Check sheet for the drawn part. Datum: minimum x, y, z corner. Units: mm. A direction names the side the tool comes from. Round coordinates to 2 decimals unless told otherwise and drop trailing zeros. Write each loop counter-clockwise with the first axis right and the second up, starting at its lowest first coordinate (ties: lowest second). Pieces come first, ordered by that corner, then holes. Notation, with made-up numbers: (67, -29) -> (114, -29) arc R18 ccw to (114, 3) -> close; hole circle Ø7 at (86.25, -34). An arc over 180 degrees is marked (long way). Use CSV: the item, a comma, the result in double quotes.
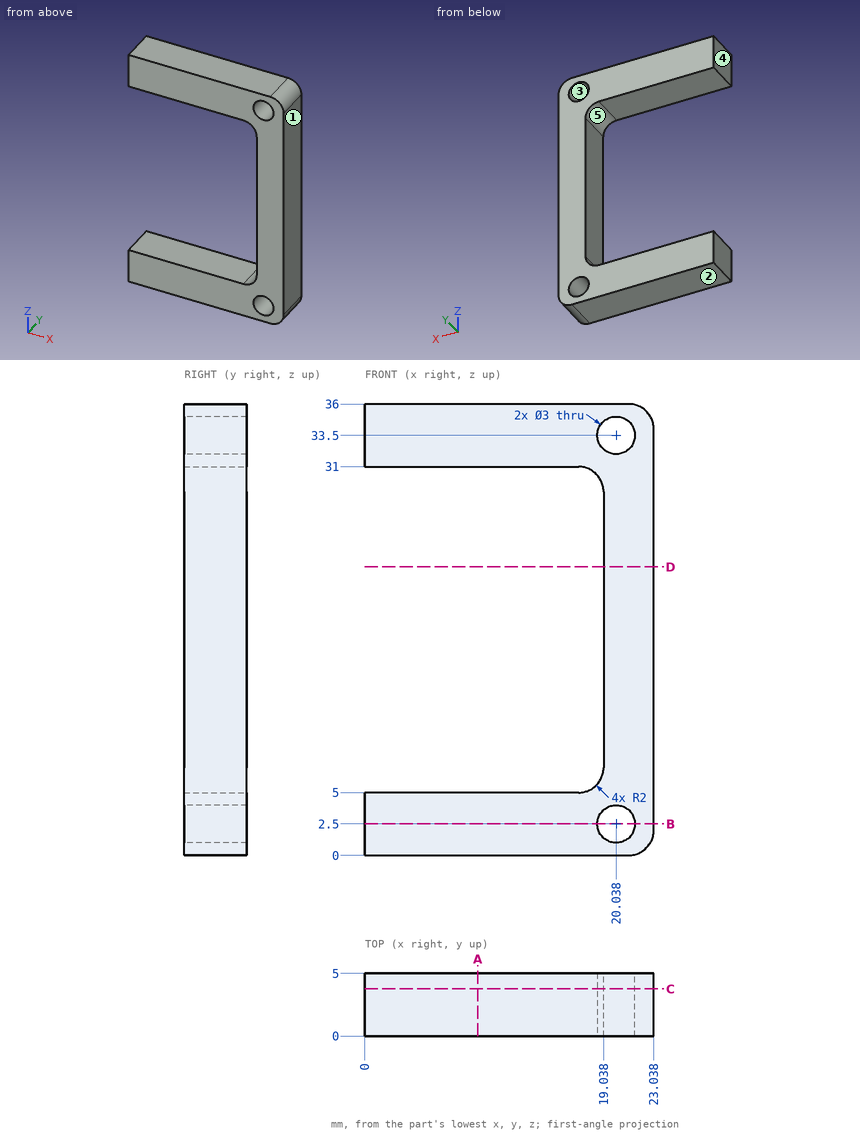
Q1. Section check B-B (z = 2.5). Record the cut outline in (x, y), plus the area to 3 significant figures.
Filled in:
outline,"(0, 0) -> (18.54, 0) -> (18.54, 5) -> (0, 5) -> close; (21.54, 0) -> (23.04, 0) -> (23.04, 5) -> (21.54, 5) -> close"
area,"100 mm²"
Q2. Section check C-C (y = 3.75). Record the cut outline in (x, z).
Filled in:
outline,"(0, 0) -> (21.04, 0) arc R2 ccw to (23.04, 2) -> (23.04, 34) arc R2 ccw to (21.04, 36) -> (0, 36) -> (0, 31) -> (17.04, 31) arc R2 cw to (19.04, 29) -> (19.04, 7) arc R2 cw to (17.04, 5) -> (0, 5) -> close; hole circle Ø3 at (20.04, 2.5); hole circle Ø3 at (20.04, 33.5)"
Q3. Section check D-D (z = 23). Record the cut outline in (x, y), plus the area to 3 significant figures.
Filled in:
outline,"(19.04, 0) -> (23.04, 0) -> (23.04, 5) -> (19.04, 5) -> close"
area,"20.0 mm²"
Q4. Go/stop test with flat-tipped pins: P1, Ø2.5, axis at x = 20.04, z = 33.5, coming from the -Y side; P2, Ø1.5, axis at y = 2, z = 23, coming from the -X side. Record where each tip stops, or that it passes through.
Filled in:
P1,"through"
P2,"x = 19.04"
Q5. Material ranges on L1, parallel to Z at x = 11.25, y = 3.7; L2, parallel to X at y = 1.5, z = 33.5; L3, parallel to Z at x = 19.25, y = 3.4 (1 decimal), recorded low to high.
Filled in:
L1,"0 to 5, 31 to 36"
L2,"0 to 18.54, 21.54 to 23.04"
L3,"0 to 1.2, 3.8 to 32.2, 34.8 to 36"
Q6. Access from +Z, -Z, +X, -X, +Y, -Y to the whole of each face (thin tool, end or side, straight path). Record for the marked faces 4 and 5.
Filled in:
face 4,"+Z, -Z, -X, +Y, -Y"
face 5,"-X, +Y, -Y"
Q7. Mould release check, pull along Z, two halves, no side actions. Record for the marked faces 1, 2 and 3: released by +Z, released by -Z, zero draft, split by the parting line, or undercut.
Filled in:
face 1,"zero draft"
face 2,"released by -Z"
face 3,"undercut"
Q8. Section check A-A (x = 9). Record the cut outline in (y, z).
Filled in:
outline,"(0, 0) -> (5, 0) -> (5, 5) -> (0, 5) -> close; (0, 31) -> (5, 31) -> (5, 36) -> (0, 36) -> close"
